Autodesk Inventor part; units mm, degrees
ref_plane "YZ Plane" through (0, 0, 0) normal (1, 0, 0) x (0, 1, 0)
ref_plane "XZ Plane" through (0, 0, 0) normal (0, 1, 0) x (-1, 0, 0)
ref_plane "XY Plane" through (0, 0, 0) normal (0, 0, 1) x (1, 0, 0)
sketch "Sketch1" plane through (0, 0, 0) normal (0, 1, 0) x (-1, 0, 0)
  line L0 (0, 0) -> (6, 0)
  line L1 (6, 0) -> (6, -82)
  line L2 (6, -82) -> (0, -82)
  line L3 (0, -82) -> (0, 0)
  circle A0 centre (3, -3) radius 1
  circle A1 centre (3, -79) radius 1
  circle A2 centre (3, -41) radius 1
  point P0 (3, 0)
  point P1 (6, -41)
  dimension "d0" = 6
  dimension "d1" = 82
  dimension "d2" = 2
  dimension "d3" = 2
  dimension "d4" = 76
  dimension "d5" = 3
  dimension "d6" = 3
  dimension "d7" = 3
  dimension "d11" = 2
  dimension "d12" = 3
  dimension "d13" = 41
extrude "Extrusion1" add sketch "Sketch1" along normal blind 3
fillet "Fillet1" radius 2 4 edges at (0, 1.5, 0) (-6, 1.5, 0) (0, 1.5, -82) (-6, 1.5, -82)
equation "\"d6\" = 0.5 * d0"
equation "\"d7\" = d6"
equation "\"d13\" = 0.5 * d1"
properties part number "Steering_Linkage"
Check sheet for the modelled part. Datum: model origin and axes. Units: mm. Round coordinates to 2 decimals unless told otherwise and drop trailing zeros. Write each loop counter-clockwise with the first axis right and the second up, starting at its lowest first coordinate (ties: lowest second). Pieces come first, ordered by that corner, then holes. Notation, with made-up numbers: (82, 61) -> (114, 61) arc R23 ccw to (114, 70) -> close; hole circle Ø7 at (-32, 30). An arc over 180 degrees is marked (long way). Put each result on its own line as item: value.
(1) Sectioned sample at B-B (y = 1.4). Enter the section's corners in (x, z).
Values found:
outline: (-6, -80) arc R2 ccw to (-4, -82) -> (-2, -82) arc R2 ccw to (0, -80) -> (0, -2) arc R2 ccw to (-2, 0) -> (-4, 0) arc R2 ccw to (-6, -2) -> close; hole circle Ø2 at (-3, -79); hole circle Ø2 at (-3, -41); hole circle Ø2 at (-3, -3)
(2) Sectioned sample at A-A (x = -3). Enter the section's corners in (y, z), plus the area to 3 significant figures.
Values found:
outline: (0, -82) -> (3, -82) -> (3, -80) -> (0, -80) -> close; (0, -78) -> (3, -78) -> (3, -42) -> (0, -42) -> close; (0, -40) -> (3, -40) -> (3, -4) -> (0, -4) -> close; (0, -2) -> (3, -2) -> (3, 0) -> (0, 0) -> close
area: 228 mm^2
(3) Material ranges on line 1 (Z direction, x = -3, y = 2.3); line 2 (X direction, y = 1.65, z = -79); line 3 (Z direction, x = -1.9, y = 2.3), recorded low to high.
Values found:
line 1: z = -82 to -80, -78 to -42, -40 to -4, -2 to 0
line 2: x = -6 to -4, -2 to 0
line 3: z = -82 to 0
(4) Mould release check, pull along X, two halves, no side actions. Record for faces 1 (the face through (-5.4, 1.52, -81.43)), 2 (the face through (-3, 1, 0)), 3 (the face through (-3, 1, -42)): released by +X, released by -X, zero draft, split by the parting line, or undercut.
Values found:
face 1: released by -X
face 2: zero draft
face 3: undercut
(5) Sectioned sample at C-C (z = -79). Enter the section's corners in (x, y), plus the area to 3 significant figures.
Values found:
outline: (-6, 0) -> (-4, 0) -> (-4, 3) -> (-6, 3) -> close; (-2, 0) -> (0, 0) -> (0, 3) -> (-2, 3) -> close
area: 12.0 mm^2
